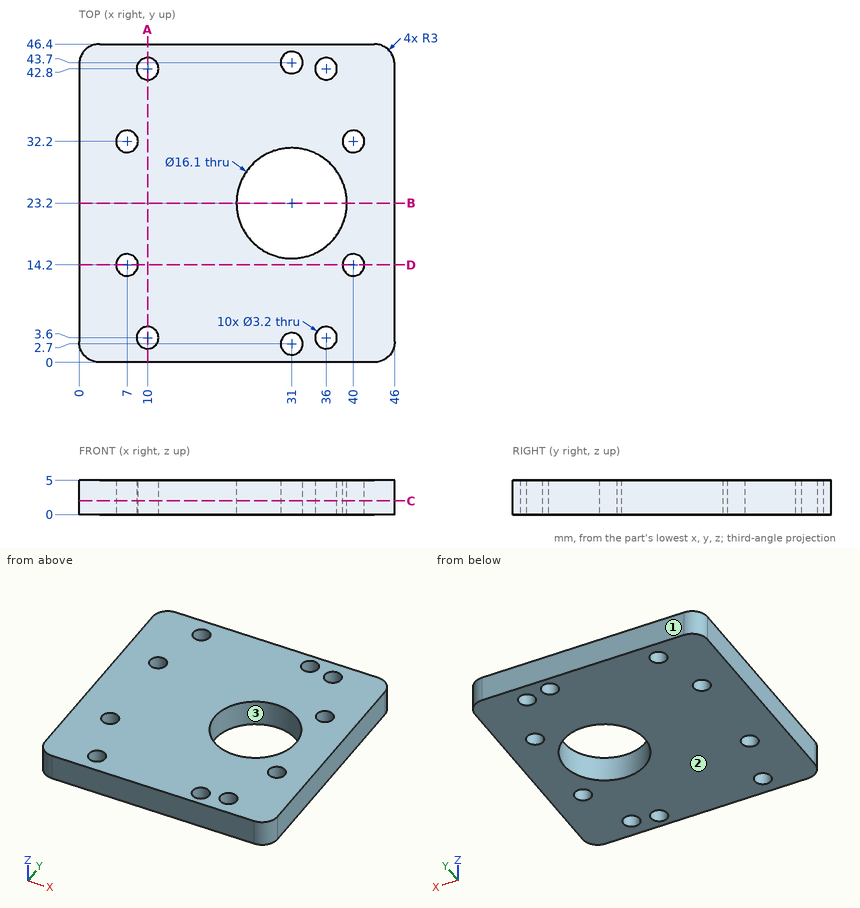
Print and shaded views of the part. All mm, measured from the part's lowest x, y and z. Coordinates: 2 decimals unless noted, no trailing zeros. Order: outer loops, then holes, each group sorted by start corner. A loop starts at its lowest first (then second) coordinate and runs counter-clockwise, first axis right, second up. Notation, with made-up numbers: (21, 33.25) - (56, 33.25) arc R19 ccw to (56, 41.25) - close; hole circle Ø2 at (55, 25). An arc over 180 degrees is marked (long way). Return JSON: item names as keys, results as strings. Group by question number.
Item 1: Cut at C-C (z = 2). State how many separate pieces and enclosed holes the cut face has, plus the area to 3 significant figures.
Item 2: Pull direction Y, two halves, no side cores. Call the marked faces 1, 2 and 3: pulls with the +Y half, pulls with the -Y half, needs draft (parallel to the pull), parting line crosses it, or undercut.
Item 3: Cut at B-B (y = 23.2). List the corners of the cut face in (x, z), plus the area to 4 significant figures.
Item 4: Cut at A-A (x = 10). List the corners of the cut face in (y, z), plus the area to 3 significant figures.
Item 5: Drill centre lines: probe 1 along Y at (x, z) = (31, 3.95); probe 2 along Y at (x, z) = (40, 2.95); probe 3 along Y at (x, z) = (10, 1.5). Where is each one in solid material? Low to high. Write a range as from..to.
Item 6: Cut at D-D (y = 14.2). List the corners of the cut face in (x, z).
Item 7: Pin check, flat tip, straight feed: pin 1 (2.5 mm diameter, centred on x = 36, y = 42.8, fed in from +Z). Stop position of the tip, or through.
Check values:
{
 "1": {"separate pieces": "1", "enclosed holes": "11", "area": "1,840 mm2"},
 "2": {"face 1": "pulls with the +Y half", "face 2": "needs draft", "face 3": "undercut"},
 "3": {"outline": "(0, 0) - (22.95, 0) - (22.95, 5) - (0, 5) - close; (39.05, 0) - (46, 0) - (46, 5) - (39.05, 5) - close", "area": "149.5 mm2"},
 "4": {"outline": "(0, 0) - (2, 0) - (2, 5) - (0, 5) - close; (5.2, 0) - (41.2, 0) - (41.2, 5) - (5.2, 5) - close; (44.4, 0) - (46.4, 0) - (46.4, 5) - (44.4, 5) - close", "area": "200 mm2"},
 "5": {"probe 1": "y = 0..1.1, 4.3..15.15, 31.25..42.1, 45.3..46.4", "probe 2": "y = 0..12.6, 15.8..30.6, 33.8..46.4", "probe 3": "y = 0..2, 5.2..41.2, 44.4..46.4"},
 "6": {"outline": "(0, 0) - (5.4, 0) - (5.4, 5) - (0, 5) - close; (8.6, 0) - (38.4, 0) - (38.4, 5) - (8.6, 5) - close; (41.6, 0) - (46, 0) - (46, 5) - (41.6, 5) - close"},
 "7": {"pin 1": "passes through"}
}
